Verification items for the finished model (mm, model axes). Coordinates: 2 decimals unless noted, no trailing zeros. Order: outer loops, then holes, each group sorted by start corner. A loop starts at its lowest first (then second) coordinate and runs counter-clockwise, first axis right, second up. Notation, with made-up numbers: M -7.75,33.5 L 13.25,33.5 A29 cw 13.25,54.5 Z; hole C 1.25,42.5 d4. An arc over 180 degrees is marked long. Return JSON: item names as keys, results as strings. Group by question number.
Q1. Thickness scan on probe 1 along Y at (x, z) = (-13, 163); probe 2 along X at (y, z) = (-19.1, 175); probe 3 along Z at (x, y) = (-14, -17.5). Record the ranges inside material, lowest first.
Q2. Section check A-A, the plane y = 0. Enter the section's corners in (x, z).
Q3. Go/stop test with flat-tipped pins: pin 1 Ø6.5 at (x, y) = (13.5, 13.5) entering from +Z; pin 2 Ø4 at (x, z) = (0.5, 174) entering from +Y; pin 3 Ø5 at (y, z) = (-3, 168) entering from -X; pin 4 Ø1 at (y, z) = (2.5, 124) entering from +X. Record where each tip stops, or that it passes through.
Q4. Section check C-C, the plane z = 154.5. Count the separate pieces of the cut face and the enclosed holes in it, then the cut area to 3 significant figures.
from build123d import *

# Parameters (mm, degrees)
SKETCH_1_W                  = 40
SKETCH_1_H                  = 40
EXTRUDE_1_DEPTH             = 320
SKETCH_2_R                  = 3.25
SKETCH_2_R_2                = 4
CUT_EXTRUDE_1_DEPTH         = 321
HOLE_WIZARD_3_5_3_5_1_D     = 3.5
HOLE_WIZARD_3_5_3_5_1_DEPTH = 7.5
HOLE_WIZARD_3_5_3_5_1_TIP   = 1.051506083


with BuildPart() as part:
    # 草圖1 → 伸長1 (new body)
    with BuildSketch(Plane.XY):
        Rectangle(SKETCH_1_W, SKETCH_1_H)
    extrude(amount=EXTRUDE_1_DEPTH)

    # 草圖2 → 除料-伸長1 (cut, through all)
    with BuildSketch(Plane(origin=(0, 0, 0), x_dir=(-1, 0, 0), z_dir=(0, 0, -1))):
        Circle(SKETCH_2_R)
        with Locations((-13.5, 13.5)):
            Circle(SKETCH_2_R_2)
        with Locations((13.5, 13.5)):
            Circle(SKETCH_2_R_2)
        with Locations((-13.5, -13.5)):
            Circle(SKETCH_2_R_2)
        with Locations((13.5, -13.5)):
            Circle(SKETCH_2_R_2)
        with BuildLine():
            Line((5, 14.5), (7.5, 14.5))
            Line((7.5, 14.5), (7.5, 13.5))
            ThreePointArc((7.5, 13.5), (0, 6), (-7.5, 13.5))
            Line((-7.5, 13.5), (-7.5, 14.5))
            Line((-7.5, 14.5), (-5, 14.5))
            Line((-5, 14.5), (-5, 20))
            Line((-5, 20), (5, 20))
            Line((5, 20), (5, 14.5))
        make_face()
        with BuildLine():
            Line((14.5, -5), (14.5, -7.5))
            Line((14.5, -7.5), (13.5, -7.5))
            ThreePointArc((13.5, -7.5), (6, 0), (13.5, 7.5))
            Line((13.5, 7.5), (14.5, 7.5))
            Line((14.5, 7.5), (14.5, 5))
            Line((14.5, 5), (20, 5))
            Line((20, 5), (20, -5))
            Line((20, -5), (14.5, -5))
        make_face()
        with BuildLine():
            Line((-5, -14.5), (-7.5, -14.5))
            Line((-7.5, -14.5), (-7.5, -13.5))
            ThreePointArc((-7.5, -13.5), (0, -6), (7.5, -13.5))
            Line((7.5, -13.5), (7.5, -14.5))
            Line((7.5, -14.5), (5, -14.5))
            Line((5, -14.5), (5, -20))
            Line((5, -20), (-5, -20))
            Line((-5, -20), (-5, -14.5))
        make_face()
        with BuildLine():
            Line((-14.5, 5), (-14.5, 7.5))
            Line((-14.5, 7.5), (-13.5, 7.5))
            ThreePointArc((-13.5, 7.5), (-6, 0), (-13.5, -7.5))
            Line((-13.5, -7.5), (-14.5, -7.5))
            Line((-14.5, -7.5), (-14.5, -5))
            Line((-14.5, -5), (-20, -5))
            Line((-20, -5), (-20, 5))
            Line((-20, 5), (-14.5, 5))
        make_face()
    extrude(amount=-CUT_EXTRUDE_1_DEPTH, mode=Mode.SUBTRACT)

    # Ø3.5 (3.5) 直徑孔1
    with Locations(Plane(origin=(0, -20, 0), x_dir=(-1, 0, 0), z_dir=(0, -1, 0))):
        with Locations((-16, -145), (-16, -175), (14, -145), (14, -175)):
            Hole(HOLE_WIZARD_3_5_3_5_1_D / 2, depth=HOLE_WIZARD_3_5_3_5_1_DEPTH)
            with Locations((0, 0, -(HOLE_WIZARD_3_5_3_5_1_DEPTH + HOLE_WIZARD_3_5_3_5_1_TIP / 2))):  # 118° drill point
                Cone(0, HOLE_WIZARD_3_5_3_5_1_D / 2, HOLE_WIZARD_3_5_3_5_1_TIP, mode=Mode.SUBTRACT)


solid = part.part
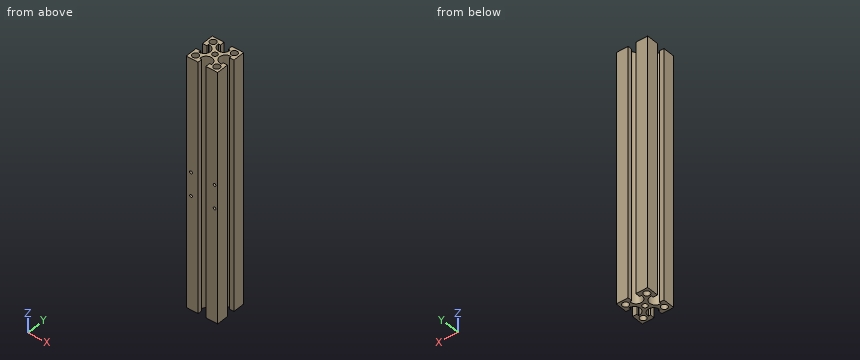
Numbers:
{
 "1": {"probe 1": "y = -20 to -17.47, -9.53 to -7.48, 7.48 to 9.53, 17.47 to 20", "probe 2": "x = -20 to -15.75, -12.25 to -5, 5 to 14.25, 17.75 to 20", "probe 3": "z = 0 to 143.25, 146.75 to 173.25, 176.75 to 320"},
 "2": {"outline": "M -6,0 L -3.25,0 L -3.25,320 L -6,320 Z; M 3.25,0 L 6,0 L 6,320 L 3.25,320 Z"},
 "3": {"pin 1": "passes through", "pin 2": "stops at y = 6.43", "pin 3": "stops at x = -20", "pin 4": "stops at x = 6.63"},
 "4": {"separate pieces": "1", "enclosed holes": "5", "area": "732 mm2"}
}
